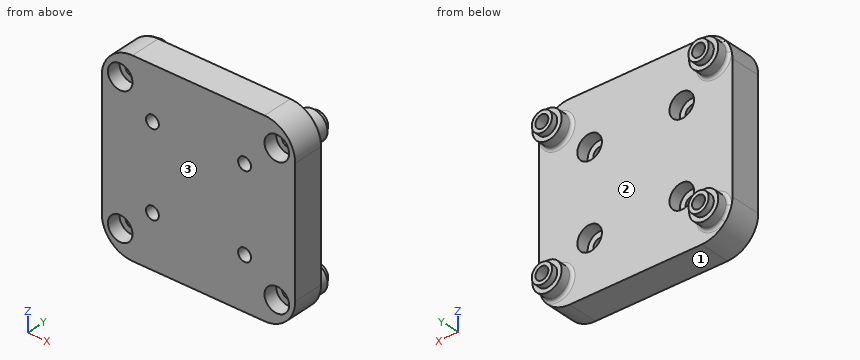
```python
from build123d import *

# Parameters (mm, degrees)
ESQUISSE1_W             = 63
ESQUISSE1_H             = 61
BOSS_EXTRU_1_DEPTH      = 10
ESQUISSE4_R             = 4.75
BOSS_EXTRU_3_DEPTH      = 4
ESQUISSE5_R             = 3.3
BOSS_EXTRU_4_DEPTH      = 2
ESQUISSE6_R             = 2.1
ENL_V_MAT_EXTRU_2_DEPTH = 90.140338792
CONG_1_R                = 10
CONG_2_R                = 1
ESQUISSE7_R             = 2.1
ENL_V_MAT_EXTRU_3_DEPTH = 90.140338931
ESQUISSE8_R             = 4
ENL_V_MAT_EXTRU_4_DEPTH = 4
ESQUISSE9_R             = 4
ENL_V_MAT_EXTRU_5_DEPTH = 4.5


with BuildPart() as part:
    # Esquisse1 → Boss.-Extru.1 (new body)
    with BuildSketch(Plane(origin=(0, 0, 0), x_dir=(1, 0, 0), z_dir=(0, 1, 0))):
        with Locations((31.5, 30.5)):
            Rectangle(ESQUISSE1_W, ESQUISSE1_H)
    extrude(amount=BOSS_EXTRU_1_DEPTH)

    # Esquisse4 → Boss.-Extru.3 (add)
    with BuildSketch(Plane(origin=(0, 10, 0), x_dir=(1, 0, 0), z_dir=(0, 1, 0))):
        with Locations(Location((6, 8, 0), (0, 0, 90))):
            Circle(ESQUISSE4_R)
        with Locations(Location((6, 53, 0), (0, 0, 90))):
            Circle(ESQUISSE4_R)
        with Locations(Location((57, 8, 0), (0, 0, 90))):
            Circle(ESQUISSE4_R)
        with Locations(Location((57, 53, 0), (0, 0, 90))):
            Circle(ESQUISSE4_R)
    extrude(amount=BOSS_EXTRU_3_DEPTH)

    # Esquisse5 → Boss.-Extru.4 (add)
    with BuildSketch(Plane(origin=(0, 14, 0), x_dir=(1, 0, 0), z_dir=(0, 1, 0))):
        with Locations(Location((57, 53, 0), (0, 0, 270))):
            Circle(ESQUISSE5_R)
        with Locations(Location((57, 8, 0), (0, 0, 270))):
            Circle(ESQUISSE5_R)
        with Locations(Location((6, 8, 0), (0, 0, 270))):
            Circle(ESQUISSE5_R)
        with Locations(Location((6, 53, 0), (0, 0, 270))):
            Circle(ESQUISSE5_R)
    extrude(amount=BOSS_EXTRU_4_DEPTH)

    # Esquisse6 → Enlèv. mat.-Extru.2 (cut, through all)
    with BuildSketch(Plane(origin=(0, 16, 0), x_dir=(1, 0, 0), z_dir=(0, 1, 0))):
        with Locations(Location((6, 8, 0), (0, 0, 270))):
            Circle(ESQUISSE6_R)
        with Locations(Location((6, 53, 0), (0, 0, 270))):
            Circle(ESQUISSE6_R)
        with Locations(Location((57, 53, 0), (0, 0, 270))):
            Circle(ESQUISSE6_R)
        with Locations(Location((57, 8, 0), (0, 0, 270))):
            Circle(ESQUISSE6_R)
    extrude(amount=-ENL_V_MAT_EXTRU_2_DEPTH, mode=Mode.SUBTRACT)

    # Congé1
    cong_1_edges = [part.edges().sort_by_distance(p)[0] for p in [
        (0, 5, -61),
        (63, 5, -61),
        (63, 5, 0),
        (0, 5, 0),
    ]]
    fillet(cong_1_edges, radius=CONG_1_R)

    # Congé2
    cong_2_edges = [part.edges().sort_by_distance(p)[0] for p in [
        (6, 10, -3.25),
        (6, 10, -48.25),
        (57, 10, -3.25),
        (57, 10, -48.25),
    ]]
    fillet(cong_2_edges, radius=CONG_2_R)

    # Esquisse7 → Enlèv. mat.-Extru.3 (cut, through all)
    with BuildSketch(Plane(origin=(0, 0, 0), x_dir=(-1, 0, 0), z_dir=(0, -1, 0))):
        with Locations(Location((-16.5, 17, 0), (0, 0, 90))):
            Circle(ESQUISSE7_R)
        with Locations(Location((-46.5, 17, 0), (0, 0, 90))):
            Circle(ESQUISSE7_R)
        with Locations(Location((-16.5, 44, 0), (0, 0, 90))):
            Circle(ESQUISSE7_R)
        with Locations(Location((-46.5, 44, 0), (0, 0, 90))):
            Circle(ESQUISSE7_R)
    extrude(amount=-ENL_V_MAT_EXTRU_3_DEPTH, mode=Mode.SUBTRACT)

    # Esquisse8 → Enlèv. mat.-Extru.4 (cut)
    with BuildSketch(Plane(origin=(0, 10, 0), x_dir=(1, 0, 0), z_dir=(0, 1, 0))):
        with Locations(Location((16.5, 44, 0), (0, 0, 270))):
            Circle(ESQUISSE8_R)
        with Locations(Location((46.5, 44, 0), (0, 0, 270))):
            Circle(ESQUISSE8_R)
        with Locations(Location((46.5, 17, 0), (0, 0, 270))):
            Circle(ESQUISSE8_R)
        with Locations(Location((16.5, 17, 0), (0, 0, 270))):
            Circle(ESQUISSE8_R)
    extrude(amount=-ENL_V_MAT_EXTRU_4_DEPTH, mode=Mode.SUBTRACT)

    # Esquisse9 → Enlèv. mat.-Extru.5 (cut)
    with BuildSketch(Plane(origin=(0, 0, 0), x_dir=(-1, 0, 0), z_dir=(0, -1, 0))):
        with Locations(Location((-57, 8, 0), (0, 0, 90))):
            Circle(ESQUISSE9_R)
        with Locations(Location((-57, 53, 0), (0, 0, 90))):
            Circle(ESQUISSE9_R)
        with Locations(Location((-6, 53, 0), (0, 0, 90))):
            Circle(ESQUISSE9_R)
        with Locations(Location((-6, 8, 0), (0, 0, 90))):
            Circle(ESQUISSE9_R)
    extrude(amount=-ENL_V_MAT_EXTRU_5_DEPTH, mode=Mode.SUBTRACT)


solid = part.part
```
Design review of the part built by this model. Coordinates are the model's own, in mm. Face numbers are marked on the shaded views. Round coordinates to 2 decimals unless told otherwise and drop trailing zeros. Write each loop counter-clockwise with the first axis right and the second up, starting at its lowest first coordinate (ties: lowest second). Pieces come first, ordered by that corner, then holes. Notation, with made-up numbers: (-38, 79.25) -> (-24, 79.25) arc R15 cw to (-24, 83.25) -> close; hole circle Ø10 at (-18, 63.25). An arc over 180 degrees is marked (long way). Write item = value, one per line. Start each with the question number.
1) Take a section at B-B, the plane z = -17. State the section outline as (x, y) points, plus the area to 3 significant figures.
2) Wall thickness on probe 1 along X at (y, z) = (12.5, -8); probe 2 along X at (y, z) = (2.85, -44); probe 3 along X at (y, z) = (2.1, -53): over which ranges is each line inside the solid? List them lowest first. Write a range as from..to.
3) Clearance check with flat-ended pins moving along their axes: pin 1 (13 mm diameter, centred on x = 16.5, z = -17, fed in from +Y); pin 2 (4 mm diameter, centred on x = 5.5, z = -8.5, fed in from -Y); pin 3 (1.5 mm diameter, centred on y = 11.5, z = -8, fed in from -X); pin 4 (9 mm diameter, centred on x = 57, z = -8, fed in from +Y). State where each tip first meets the part, or that it passes through.
4) Take a section at D-D, the plane y = 5.25. Count the separate pieces of the cut face and the enclosed holes in it, plus the area to 3 significant figures.
5) Take a section at A-A, the plane y = 12. State the section outline as (x, z) points.
6) Take a section at C-C, the plane x = 46.5. State the section outline as (y, z) points, plus the area to 3 significant figures.
7) Mouldability with a two-part tool opening along Z and no side actions: class the marked faces 1, 2 and 3 as +Z half, -Z half, draft (parallel to the pull), parting line (faces both ways), or undercut.
Results list:
q1.outline = (0, 0) -> (14.4, 0) -> (14.4, 6) -> (12.5, 6) -> (12.5, 10) -> (0, 10) -> close; (18.6, 0) -> (44.4, 0) -> (44.4, 6) -> (42.5, 6) -> (42.5, 10) -> (20.5, 10) -> (20.5, 6) -> (18.6, 6) -> close; (48.6, 0) -> (63, 0) -> (63, 10) -> (50.5, 10) -> (50.5, 6) -> (48.6, 6) -> close
q1.area = 516 mm²
q2.probe_1 = 1.25..3.9, 8.1..10.75, 52.25..54.9, 59.1..61.75
q2.probe_2 = 0..14.4, 18.6..44.4, 48.6..63
q2.probe_3 = 0.2..2, 10..53, 61..62.8
q3.pin_1 = 10
q3.pin_2 = 4.5
q3.pin_3 = 1.22
q3.pin_4 = 16
q4.separate_pieces = 1
q4.enclosed_holes = 8
q4.area = 3,650 mm²
q5.outline = circle Ø9.5 at (6, -53); circle Ø9.5 at (6, -8); circle Ø9.5 at (57, -53); circle Ø9.5 at (57, -8); hole circle Ø4.2 at (6, -53); hole circle Ø4.2 at (6, -8); hole circle Ø4.2 at (57, -53); hole circle Ø4.2 at (57, -8)
q6.outline = (0, -61) -> (10, -61) -> (10, -48) -> (6, -48) -> (6, -46.1) -> (0, -46.1) -> close; (0, -41.9) -> (6, -41.9) -> (6, -40) -> (10, -40) -> (10, -21) -> (6, -21) -> (6, -19.1) -> (0, -19.1) -> close; (0, -14.9) -> (6, -14.9) -> (6, -13) -> (10, -13) -> (10, 0) -> (0, 0) -> close
q6.area = 496 mm²
q7.face_1 = -Z half
q7.face_2 = undercut
q7.face_3 = draft
